Can you work these out from the model? Positions are in its coordinate system, mm. Give positions to 0.01 mm unless a question says otherwise; leave off trailing zeros. Write each loop counter-clockwise with the first axis right and the second up, starting at its lowest first coordinate (ties: lowest second). Pieces come first, ordered by that corner, then holes.
Autodesk Inventor part; units mm, degrees
ref_plane "YZ Plane" through (0, 0, 0) normal (1, 0, 0) x (0, 1, 0)
ref_plane "XZ Plane" through (0, 0, 0) normal (0, 1, 0) x (-1, 0, 0)
ref_plane "XY Plane" through (0, 0, 0) normal (0, 0, 1) x (1, 0, 0)
sketch "Sketch1" plane through (0, 0, 0) normal (0, 0, 1) x (1, 0, 0)
  circle A0 centre (0, 0) radius 2
  dimension "d0" = 4
extrude "Extrusion1" add sketch "Sketch1" along normal blind 5.7
sketch "Sketch2" plane through (0, 0, 5.7) normal (0, 0, 1) x (1, 0, 0)
  circle A0 centre (0, 0) radius 2
  circle A1 centre (0, 2) radius 0.1621
extrude "Extrusion2" add sketch "Sketch2" against normal blind 5.7 contours A1 A0 | A0 A1 picked at (0, 1.9455) picked at (0.0067, 2.0531)
pattern_circular "Circular Pattern1" count 24 over 360 about axis through (0, 0, -10) along (0, 0, 1) of "Extrusion2"
sketch "Sketch3" plane through (0, 0, 5.7) normal (0, 0, 1) x (1, 0, 0)
  point P0 (0, 0)
  point P1 (0, 0)
hole "Hole1" at (0, 0, 5.7) direction (0, 0, -1) diameter 3 end through all
thread "Thread1"
properties part number "M3ThreadedInsert"
(1) Imagine slicing it at B-B, the plane x = 1. Write out the boundary of the cut face in (y, z), plus the area to 3 significant figures.
Returned:
outline: (-1.89, 0) - (-1.12, 0) - (-1.12, 5.7) - (-1.89, 5.7) - close; (1.12, 0) - (1.89, 0) - (1.89, 5.7) - (1.12, 5.7) - close
area: 8.85 mm2
(2) Will these pins go through, and if not, where does the flat tip stop? P1, Ø1.5, axis at x = -1, z = 4.5, coming from the +Y side; P2, Ø1, axis at y = 1, z = 3, coming from the -X side.
Returned:
P1: stops at y = 2.09
P2: stops at x = -2.09
(3) Imagine slicing it at A-A, the plane y = 0. Write out the boundary of the cut face in (x, z), plus the area to 3 significant figures.
Returned:
outline: (-2.16, 0) - (-1.5, 0) - (-1.5, 5.7) - (-2.16, 5.7) - close; (1.5, 0) - (2.16, 0) - (2.16, 5.7) - (1.5, 5.7) - close
area: 7.55 mm2
(4) If I drill on L1, parallel to X at y = 0, z = 2.9; L2, parallel to X at y = -0.3, z = 4.9, over which ranges is the centre line in solid material (lowest first)?
Returned:
L1: x = -2.16 to -1.5, 1.5 to 2.16
L2: x = -1.98 to -1.47, 1.47 to 1.98
